Autodesk Inventor part; units mm, degrees
ref_plane "YZ Plane" through (0, 0, 0) normal (1, 0, 0) x (0, 1, 0)
ref_plane "XZ Plane" through (0, 0, 0) normal (0, 1, 0) x (-1, 0, 0)
ref_plane "XY Plane" through (0, 0, 0) normal (0, 0, 1) x (1, 0, 0)
sketch "Sketch1" plane through (0, 0, 0) normal (0, 1, 0) x (-1, 0, 0)
  circle A0 centre (0, 0) radius 2.3241
  line L0 (0, 0) -> (0, -63.5)
  circle A1 centre (0, -63.5) radius 2.3241
  line L1 (0, 0) -> (0, -63.5) construction
  line L2 (-6.35, 0) -> (-6.35, -63.5)
  line L3 (6.35, -63.5) -> (6.35, 0)
  arc A2 (6.35, 0) -> (-6.35, 0) centre (0, 0) ccw
  arc A3 (-6.35, -63.5) -> (6.35, -63.5) centre (0, -63.5) ccw
  line L4 (0, -63.5) -> (-15.9411, -63.5) construction
  line L5 (0, -57.15) -> (-15.9411, -57.15)
  line L6 (-15.9411, -69.85) -> (0, -69.85)
  arc A4 (0, -69.85) -> (0, -57.15) centre (0, -63.5) ccw
  arc A5 (-15.9411, -57.15) -> (-15.9411, -69.85) centre (-15.9411, -63.5) ccw
  line L7 (0, -63.5) -> (-25.4, -63.5) construction
  line L8 (0, -57.15) -> (-25.4, -57.15)
  line L9 (-25.4, -69.85) -> (0, -69.85)
  arc A6 (0, -69.85) -> (0, -57.15) centre (0, -63.5) ccw
  arc A7 (-25.4, -57.15) -> (-25.4, -69.85) centre (-25.4, -63.5) ccw
  line L10 (-5.9094, 2.3241) -> (-31.2958, -61.1417)
  line L11 (-25.4, -63.5) -> (-25.4, -37.9561) construction
  line L12 (-19.05, -63.5) -> (-19.05, -37.9561)
  line L13 (-31.75, -37.9561) -> (-31.75, -63.5)
  arc A8 (-31.75, -63.5) -> (-19.05, -63.5) centre (-25.4, -63.5) ccw
  arc A9 (-19.05, -37.9561) -> (-31.75, -37.9561) centre (-25.4, -37.9561) ccw
  line L14 (-27.3182, -31.9028) -> (-18.4799, -29.102)
  point P0 (0, -31.75)
  point P1 (-7.9706, -63.5)
  point P2 (-22.0988, -61.949)
  point P3 (-12.7, -63.5)
  point P4 (-6.35, -57.15)
  point P5 (-25.4, -50.7281)
  dimension "d0" = 4.6482
  dimension "d1" = 63.5
  dimension "d2" = 4.6482
  dimension "d3" = 12.7
  dimension "d6" = 15.9411
  dimension "d7" = 25.4
extrude "Extrusion2" add sketch "Sketch1" along normal blind 1.5875 contours L5 L2 A2 L3 A4 | A4 A3 L2 L5 | L5 L8 L12 A9 L10 A2 L2 | L2 A3 L6 A5 A8 L12 L5 | A5 L12 L8 | L12 A8 A5 | A5 A8 A7 L8 L12 | L8 A7 L10 A9 L12 | L9 A8 A5
extrude "Extrusion3" add sketch "Sketch1" along normal blind 1.5875 contours L10 A9 L14 | L10 A7 L13 A9
fillet "Fillet1" radius 25.4 1 edges at (18.4799, 0.7937, -29.102)
sketch "Sketch2" plane through (0, 1.5875, 0) normal (0, 1, 0) x (1, 0, 0)
  circle A0 centre (0, 0) radius 2.3241
  line L0 (0, 0) -> (0, -25.4)
  line L1 (0, -25.4) -> (0, 0) construction
  line L2 (6.35, -25.4) -> (6.35, 0)
  line L3 (-6.35, 0) -> (-6.35, -25.4)
  arc A1 (-6.35, -25.4) -> (6.35, -25.4) centre (0, -25.4) ccw
  arc A2 (6.35, 0) -> (-6.35, 0) centre (0, 0) ccw
  circle A3 centre (0, -25.4) radius 2.3241
  line L4 (0, 0) -> (0, 12.6898)
  circle A4 centre (0, 12.6898) radius 2.3241
  point P0 (0, -12.7)
  dimension "d13" = 25.4
  dimension "d17" = 4.6482
  dimension "d20" = 4.6482
extrude "Extrusion4" add sketch "Sketch2" against normal blind 1.5875 contours A0 L0 L4 | A3 | A2 L2 A1 L3 | L4 L0 A0
fillet "Fillet2" radius 101.6 1 edges at (6.35, 0.7937, 1.2226)
extrude "Extrusion5" cut sketch "Sketch2" against normal blind 1.5875 contours A3
extrude "Extrusion6" cut sketch "Sketch2" against normal blind 1.5875 contours A4
properties part number "Lady Brown Tab Top"
Source: CAD feature listing. Evaluate the final solid. Frame: model axes, mm. Coordinates: 2 decimals unless noted, no trailing zeros. Loops run counter-clockwise (first coordinate to the right, second up) from the corner with the lowest first, then second, coordinate; pieces in that order, holes last. Notation, with made-up numbers: M 30.5,44 L 85.5,44 A23 ccw 85.5,68 Z; hole C -32.5,43 d4. An arc over 180 degrees is marked long. Answer in a Markdown table with one row per item.
Q1. Section C-C on x = 9. Return the cut outline in (y, z), plus the area to 3 significant figures.
Answers below:
| item | result |
|---|---|
| outline | M 0,-69.85 L 1.59,-69.85 L 1.59,-2.26 L 0,-2.26 Z |
| area | 107 mm^2 |
Q2. Section A-A on z = 22. Return the cut outline in (x, y), plus the area to 3 significant figures.
Answers below:
| item | result |
|---|---|
| outline | M -6.35,0 L 6.35,0 L 6.35,1.59 L -6.35,1.59 Z |
| area | 20.2 mm^2 |
Q3. Ray query, probe 1 along Z at (x, y) = (0, 0.4); probe 2 along Z at (x, y) = (1.5, 1.15); probe 3 along X at (y, z) = (0.55, 25.4). Return the intervals inside material, ascending. Write a range as from..to.
Answers below:
| item | result |
|---|---|
| probe 1 | z = -69.85..-65.82, -61.18..-15.01, -10.37..23.08, 27.72..31.75 |
| probe 2 | z = -69.85..-65.28, -61.72..-14.47, -10.91..23.62, 27.18..31.57 |
| probe 3 | x = -6.35..-2.32, 2.32..6.35 |
Q4. First-contact query: pin 1 (3 mm diameter, centred on x = 0, z = 25.4, fed in from +Y). Flat tip, straight axial feed; report the tip coordinate or a pass-through.
Answers below:
| item | result |
|---|---|
| pin 1 | passes through |
Q5. Section B-B on y = 0.6. State how many separate pieces and enclosed holes the cut face has, plus the area to 3 significant figures.
Answers below:
| item | result |
|---|---|
| separate pieces | 1 |
| enclosed holes | 3 |
| area | 2,430 mm^2 |
Q6. Draft query along X for faces 1 (the flat face through (9, 1.588, -30)), 2 (the cylindrical face through (-0.14, 0.8, 31.75)), 3 (the cylindrical face through (-0.5, 0.8, -10.42)), 4 (the cylindrical face through (8.132, 0.783, 1.841)). Return one class per face: pulls with the +X half, pulls with the -X half, needs draft (parallel to the pull), parting line crosses it, or undercut.
Answers below:
| item | result |
|---|---|
| face 1 | needs draft |
| face 2 | parting line crosses it |
| face 3 | undercut |
| face 4 | pulls with the +X half |
